Job drawing, mm, ordinate dimensions from the low corner. One solid piece. A direction names the side the tool comes from. Give positions to 0.01 mm unless a question says otherwise; leave off trailing zeros. Write each loop counter-clockwise with the first axis right and the second up, starting at its lowest first coordinate (ties: lowest second). Pieces come first, ordered by that corner, then holes. Notation, with made-up numbers: (19.5, 27) - (66.5, 27) arc R29 cw to (66.5, 62) - close; hole circle Ø11 at (63.25, 27). An arc over 180 degrees is marked (long way). Answer in a Markdown table with one row per item. Add a question column.
1. Pull direction Y, two halves, no side cores. Call the marked faces 4, 5, 6 and 7: released by +Y, released by -Y, zero draft, split by the parting line, or undercut.
2. Band-saw the part on A-A on y = 35.5. Write the cut outline in (x, z), plus the area to 3 significant figures.
3. Which spindle directions (+Z, -Z, +X, -X, +Y, -Y) get a long thin tool onto all of the face, cutting with end or side? Do the marked faces 1, 2 and 3. Say none if no direction does.
4. Drop flat-ended pins along their axis: pin 1 Ø4.5 at (x, z) = (34.5, 3.5) entering from -Y; pin 2 Ø4 at (x, y) = (30, 25) entering from +Z; pin 3 Ø1.2 at (x, z) = (5, 4.5) entering from -Y. Give the stop position or say it passes through.
5. Band-saw the part on B-B on z = 4. Write the cut outline in (x, y).
6. Band-saw the part on C-C on x = 30. Write the cut outline in (y, z).
7. Probe line 1 along X through (y, z) = (25, 1.55); line 2 along Y through (x, z) = (20, 4.45); line 3 along Z through (x, y) = (35, 3). List the from-to ranges inside material, lowest first.
8. Band-saw the part on D-D on y = 4. Write the cut outline in (x, z), plus the area to 3 significant figures.
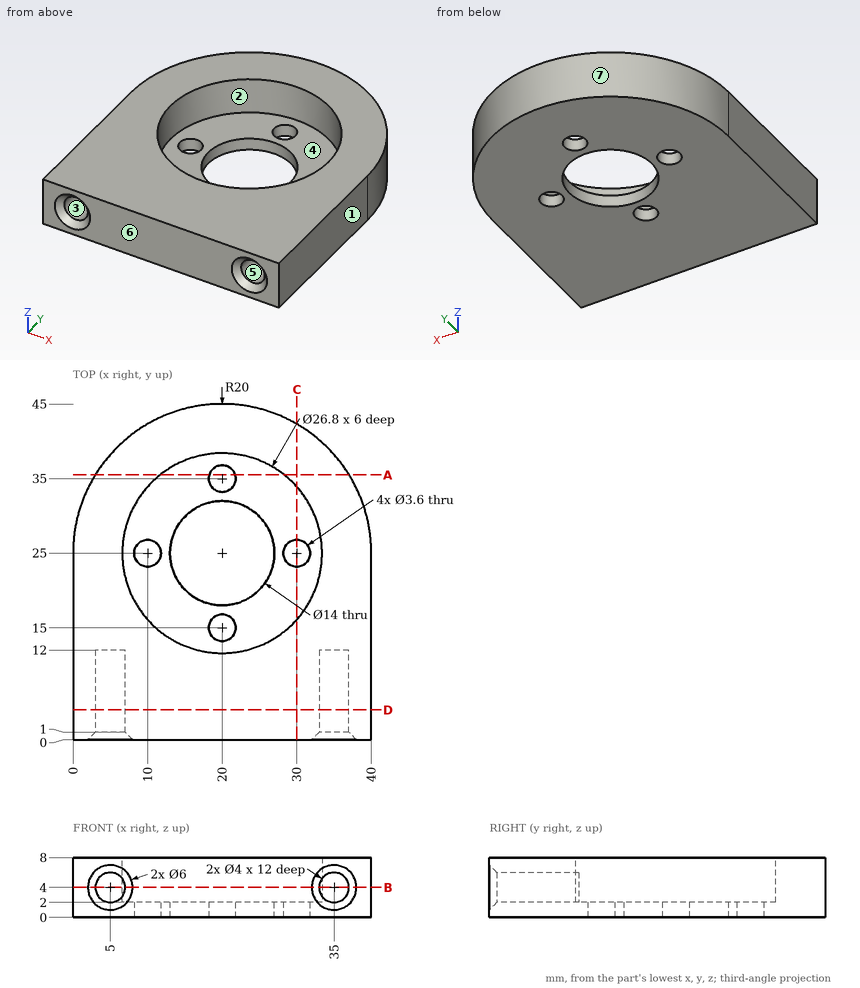
Values:
| question | item | result |
|---|---|---|
| 1 | face 4 | undercut |
| 1 | face 5 | zero draft |
| 1 | face 6 | released by -Y |
| 1 | face 7 | released by +Y |
| 2 | outline | (2.98, 0) - (18.27, 0) - (18.27, 2) - (11.67, 2) - (11.67, 8) - (2.98, 8) - close; (21.73, 0) - (37.02, 0) - (37.02, 8) - (28.33, 8) - (28.33, 2) - (21.73, 2) - close |
| 2 | area | 166 mm² |
| 3 | face 1 | +Z, -Z, +X, +Y, -Y |
| 3 | face 2 | +Z |
| 3 | face 3 | -Y |
| 4 | pin 1 | stops at y = 0.04 |
| 4 | pin 2 | stops at z = 2 |
| 4 | pin 3 | stops at y = 12 |
| 5 | outline | (0, 0) - (2, 0) - (3, 1) - (3, 12) - (7, 12) - (7, 1) - (8, 0) - (32, 0) - (33, 1) - (33, 12) - (37, 12) - (37, 1) - (38, 0) - (40, 0) - (40, 25) arc R20 ccw to (0, 25) - close; hole circle Ø26.8 at (20, 25) |
| 6 | outline | (0, 0) - (23.2, 0) - (23.2, 2) - (16.08, 2) - (16.08, 8) - (0, 8) - close; (26.8, 0) - (42.32, 0) - (42.32, 8) - (33.92, 8) - (33.92, 2) - (26.8, 2) - close |
| 7 | line 1 | x = 0 to 8.2, 11.8 to 13, 27 to 28.2, 31.8 to 40 |
| 7 | line 2 | y = 0 to 11.6, 38.4 to 45 |
| 7 | line 3 | z = 0 to 2, 6 to 8 |
| 8 | outline | (0, 0) - (40, 0) - (40, 8) - (0, 8) - close; hole circle Ø4 at (5, 4); hole circle Ø4 at (35, 4) |
| 8 | area | 295 mm² |
